```python
from build123d import *

# Parameters (mm, degrees)
SKETCH_2_W          = 80
SKETCH_2_H          = 20
SKETCH_2_R          = 2.6
EXTRUDE_1_DEPTH     = 10
SKETCH_3_W          = 30
SKETCH_3_H          = 10
CUT_EXTRUDE_1_DEPTH = 5
CHAMFER_1_SIZE      = 2


with BuildPart() as part:
    # Эскиз2 → Бобышка-Вытянуть1 (new body)
    with BuildSketch(Plane.XY):
        Rectangle(SKETCH_2_W, SKETCH_2_H)
        with Locations((-30, 0)):
            Circle(SKETCH_2_R, mode=Mode.SUBTRACT)
        with Locations((30, 0)):
            Circle(SKETCH_2_R, mode=Mode.SUBTRACT)
    extrude(amount=EXTRUDE_1_DEPTH)

    # Эскиз3 → Вырез-Вытянуть1 (cut)
    with BuildSketch(Plane(origin=(0, 0, 0), x_dir=(-1, 0, 0), z_dir=(0, 0, -1))):
        with Locations((0, -5)):
            Rectangle(SKETCH_3_W, SKETCH_3_H)
    extrude(amount=-CUT_EXTRUDE_1_DEPTH, mode=Mode.SUBTRACT)

    # Фаска1
    chamfer_1_edges = [part.edges().sort_by_distance(p)[0] for p in [
        (-40, 0, 10),
        (40, 0, 10),
    ]]
    chamfer(chamfer_1_edges, length=CHAMFER_1_SIZE)


solid = part.part
```
Source: CAD feature listing. Evaluate the final solid. Frame: model axes, mm. A direction names the side the tool comes from. Round coordinates to 2 decimals unless told otherwise and drop trailing zeros. Write each loop counter-clockwise with the first axis right and the second up, starting at its lowest first coordinate (ties: lowest second). Pieces come first, ordered by that corner, then holes. Notation, with made-up numbers: M 41,-31.5 L 64,-31.5 A36 cw 64,7.5 Z; hole C 40.25,76.25 d9. An arc over 180 degrees is marked long. Answer as a JSON object with one key per item and string values. Group by question number.
(1) Section query B-B on z = 6. Output: boundary loops of the cut face in (x, y), then the cut area to 3 significant figures.
(2) Section query A-A on x = -30. Output: boundary loops of the cut face in (y, z).
(3) Section query D-D on x = 2. Output: boundary loops of the cut face in (y, z), then the cut area to 3 significant figures.
(4) First-contact query: pin 1 (3 mm diameter, centred on x = 30, y = 0, fed in from +Z); pin 2 (11 mm diameter, centred on x = 6.5, y = -7, fed in from -Z); pin 3 (1.5 mm diameter, centred on x = 5, z = 3, fed in from -Y). Flat tips, straight axial feed; report the tip coordinate or a pass-through.
(5) Section query C-C on y = -6.5. Output: boundary loops of the cut face in (x, z), then the cut area to 3 significant figures.
(6) Reachability of faces 5 (the flat face through (0, 0, 2)), 6 (the flat face through (40, 0, 4)) from +Z, -Z, +X, -X, +Y, -Y: full face, straight path, thin tool, end or side. Return the list, or none.
(7) Ray query, line 1 (Y direction, x = -30, z = 8); line 2 (X direction, y = 0.75, z = 9); line 3 (X direction, y = -2.25, z = 8). Return the intervals inside material, ascending. Write a range as [from, to].
(8) Mould query, pull axis X, two halves, no side actions, for faces 1 (the flat face through (15, -5, 2)), 2 (the flat face through (-1, -10, 6)), 3 (the flat face through (-40, 0, 4)), 4 (the flat face through (-15, -5, 2)). Classes: +X half, -X half, draft (parallel to the pull), parting line (faces both ways), or undercut.
Computed values:
{
 "1": {"outline": "M -40,-10 L 40,-10 L 40,10 L -40,10 Z; hole C -30,0 d5.2; hole C 30,0 d5.2", "area": "1,560 mm^2"},
 "2": {"outline": "M -10,0 L -2.6,0 L -2.6,10 L -10,10 Z; M 2.6,0 L 10,0 L 10,10 L 2.6,10 Z"},
 "3": {"outline": "M -10,5 L 0,5 L 0,0 L 10,0 L 10,10 L -10,10 Z", "area": "150 mm^2"},
 "4": {"pin 1": "through", "pin 2": "z = 5", "pin 3": "y = 0"},
 "5": {"outline": "M -40,0 L -15,0 L -15,5 L 15,5 L 15,0 L 40,0 L 40,8 L 38,10 L -38,10 L -40,8 Z", "area": "646 mm^2"},
 "6": {"face 5": "-Z, -Y", "face 6": "+Z, -Z, +X, +Y, -Y"},
 "7": {"line 1": "[-10, -2.6], [2.6, 10]", "line 2": "[-39, -32.49], [-27.51, 27.51], [32.49, 39]", "line 3": "[-40, -31.3], [-28.7, 28.7], [31.3, 40]"},
 "8": {"face 1": "undercut", "face 2": "draft", "face 3": "-X half", "face 4": "undercut"}
}
